Could you check a few things on this drawing? It's one solid part, dimensions in mm from its lowest x, y, z. A direction names the side the tool comes from. Coordinates: 2 decimals unless noted, no trailing zeros. Order: outer loops, then holes, each group sorted by start corner. A loop starts at its lowest first (then second) coordinate and runs counter-clockwise, first axis right, second up. Notation, with made-up numbers: M 78.5,38 L 104.5,38 A35 ccw 104.5,77 Z; hole C 7.5,45 d8. An arc over 180 degrees is marked long. Answer as CSV lines item,"result". Start each with the question number.
1. If we section it at D-D (x = 9): List the corners of the cut face in (y, z) for me.
2. If we section it at C-C (y = 38): List the corners of the cut face in (x, z) for me, plus the area to 3 significant figures.
3. I need wall thicknesses on line 1 along Y through (x, z) = (32, 14.25); line 2 along X through (y, z) = (34.5, 12); line 3 along Y through (x, z) = (70.5, 10.75). Which ranges of each line are inside material? Lowest first, please. Write a range as from..to.
4. If we section it at A-A (x = 108): List the corners of the cut face in (y, z) for me.
5. If we section it at B-B (z = 3.75): List the corners of the cut face in (x, y) for me.
6. If we mould it in two halves opening along X, with no side actions, what happens to the marked faces 4, 5 and 6? For each: released by +X, released by -X, zero draft, split by the parting line, or undercut.
7. On a 3-axis mill with a long thin cutter (end or side, diameter ignored), from which of +Z, -Z, +X, -X, +Y, -Y can I reach the whole of each face in a straight line? I mean the marked faces 1, 2 and 3. Say none if no direction works.
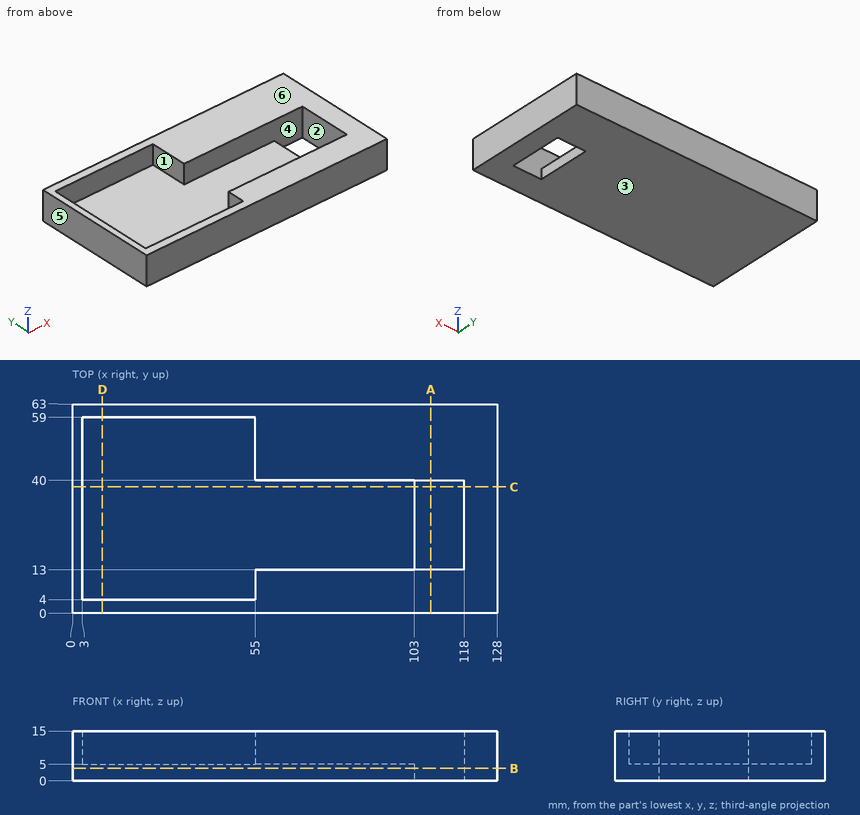
Solved:
1,outline,"M 0,0 L 63,0 L 63,15 L 59,15 L 59,5 L 4,5 L 4,15 L 0,15 Z"
2,outline,"M 0,0 L 103,0 L 103,5 L 3,5 L 3,15 L 0,15 Z; M 118,0 L 128,0 L 128,15 L 118,15 Z"
2,area,"695 mm²"
3,line 1,"0..4, 59..63"
3,line 2,"0..3, 118..128"
3,line 3,"0..13, 40..63"
4,outline,"M 0,0 L 13,0 L 13,15 L 0,15 Z; M 40,0 L 63,0 L 63,15 L 40,15 Z"
5,outline,"M 0,0 L 128,0 L 128,63 L 0,63 Z; hole M 103,13 L 118,13 L 118,40 L 103,40 Z"
6,face 4,"undercut"
6,face 5,"released by -X"
6,face 6,"zero draft"
7,face 1,"+Z"
7,face 2,"+Z, -Z"
7,face 3,"-Z, +X, -X, +Y, -Y"
